Part model, mm, in its own coordinate system. Coordinates: 2 decimals unless noted, no trailing zeros. Loops run counter-clockwise (first coordinate to the right, second up) from the corner with the lowest first, then second, coordinate; pieces in that order, holes last. Notation, with made-up numbers: M 82,-1 L 140,-1 A25 cw 140,32 Z; hole C 20.25,80.25 d5. An arc over 180 degrees is marked long. Use a Markdown table: item, result. Add a question column.
1) Wall check: probe 1 along X at (y, z) = (1.9, -43); probe 2 along X at (y, z) = (0.25, -67); probe 3 along X at (y, z) = (1.95, -62). Give the ranges that are in metal, low to high. Write a range as from..to.
2) Band-saw the part on D-D (z = -54.5). List the corners of the cut face in (x, y), plus the area to 3 significant figures.
3) Band-saw the part on A-A (z = -43). List the corners of the cut face in (x, y).
4) Pin check, flat tips, straight feed: pin 1 Ø1 at (x, z) = (-24.5, -54) entering from -Y; pin 2 Ø4 at (x, z) = (0, -65) entering from -Y. Stop position of each tip, or through.
5) Band-saw the part on C-C (y = 2.05). List the corners of the cut face in (x, z).
6) Band-saw the part on B-B (x = 0). List the corners of the cut face in (y, z), plus the area to 3 significant figures.
from build123d import *

# Parameters (mm, degrees)
BOSS_EXTRUDE1_DEPTH  = 3
CUT_EXTRUDE14_DEPTH  = 103.574363269
SKETCH14_OUTSIDE_W   = 186.736
SKETCH14_OUTSIDE_H   = 177.534
SKETCH14_OUTSIDE_W_2 = 80
SKETCH14_OUTSIDE_H_2 = 40
CUT_EXTRUDE15_DEPTH  = 103.574363269
SKETCH15_R           = 2.4
CUT_EXTRUDE16_DEPTH  = 83.856804186


with BuildPart() as part:
    # Sketch1 → Boss-Extrude1 (new body)
    with BuildSketch(Plane(origin=(0, 0, 0), x_dir=(1, 0, 0), z_dir=(0, 1, 0))):
        with BuildLine():
            ThreePointArc((36.543377003, -62.616544118), (0, 72.5), (-36.543377003, -62.616544118))
            ThreePointArc((-36.543377003, -62.616544118), (-33.085954668, -63.20954405), (-30.089832649, -61.38507948))
            ThreePointArc((-30.089832649, -61.38507948), (0, -46.75), (30.089832649, -61.38507948))
            ThreePointArc((30.089832649, -61.38507948), (33.085954668, -63.20954405), (36.543377003, -62.616544118))
        make_face()
    extrude(amount=BOSS_EXTRUDE1_DEPTH)

    # Sketch13 → Cut-Extrude14 (cut, through all)
    with BuildSketch(Plane(origin=(0, 3, 0), x_dir=(1, 0, 0), z_dir=(0, 1, 0))):
        with BuildLine():
            Line((-9.638836445, 48.2), (9.638836445, 48.2))
            ThreePointArc((9.638836445, 48.2), (10.961172041, 48.699523885), (11.622969422, 49.948571429))
            ThreePointArc((11.622969422, 49.948571429), (13.054510917, 54.765599326), (15.951885484, 58.871484058))
            ThreePointArc((15.951885484, 58.871484058), (16.449270482, 60.8240474), (14.994913363, 62.21858704))
            ThreePointArc((14.994913363, 62.21858704), (12.303854546, 62.806171379), (9.590005203, 63.277419355))
            ThreePointArc((9.590005203, 63.277419355), (8.295362524, 63.03495375), (7.432254032, 62.04))
            ThreePointArc((7.432254032, 62.04), (0, 57), (-7.432254032, 62.04))
            ThreePointArc((-7.432254032, 62.04), (-8.295362524, 63.03495375), (-9.590005203, 63.277419355))
            ThreePointArc((-9.590005203, 63.277419355), (-12.303854546, 62.806171379), (-14.994913363, 62.21858704))
            ThreePointArc((-14.994913363, 62.21858704), (-16.449270482, 60.8240474), (-15.951885484, 58.871484058))
            ThreePointArc((-15.951885484, 58.871484058), (-13.054510917, 54.765599326), (-11.622969422, 49.948571429))
            ThreePointArc((-11.622969422, 49.948571429), (-10.961172041, 48.699523885), (-9.638836445, 48.2))
        make_face()
    extrude(amount=-CUT_EXTRUDE14_DEPTH, mode=Mode.SUBTRACT)

    # Sketch14 outside → Cut-Extrude15 (cut, through all)
    with BuildSketch(Plane(origin=(0, 3, 0), x_dir=(1, 0, 0), z_dir=(0, 1, 0))):
        with Locations((0, 4.601)):
            Rectangle(SKETCH14_OUTSIDE_W, SKETCH14_OUTSIDE_H)
        with Locations((0, 57)):
            Rectangle(SKETCH14_OUTSIDE_W_2, SKETCH14_OUTSIDE_H_2, mode=Mode.SUBTRACT)
    extrude(amount=-CUT_EXTRUDE15_DEPTH, mode=Mode.SUBTRACT)

    # Sketch15 → Cut-Extrude16 (cut, through all)
    with BuildSketch(Plane(origin=(0, 3, 0), x_dir=(1, 0, 0), z_dir=(0, 1, 0))):
        with Locations(Location((0, 65, 0), (0, 0, 270))):
            Circle(SKETCH15_R)
        with Locations(Location((0, 43, 0), (0, 0, 270))):
            Circle(SKETCH15_R)
    extrude(amount=-CUT_EXTRUDE16_DEPTH, mode=Mode.SUBTRACT)


solid = part.part
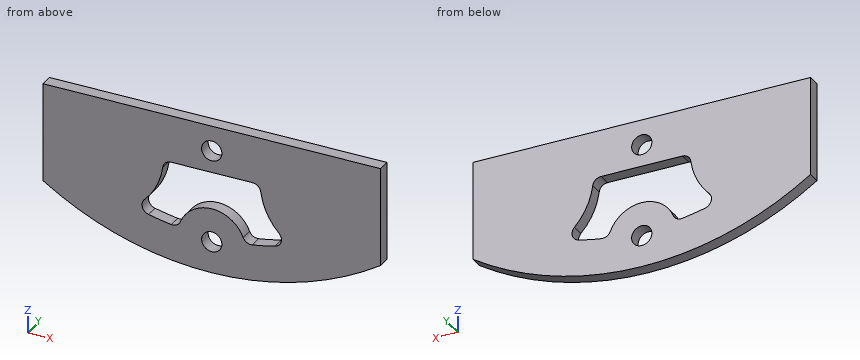
Entries:
| question | item | result |
|---|---|---|
| 1 | probe 1 | -40..-2.4, 2.4..40 |
| 1 | probe 2 | -27.7..-1.33, 1.33..27.7 |
| 1 | probe 3 | -37.58..-15.54, -7.42..7.42, 15.54..37.58 |
| 2 | outline | M -40,0 L -12.93,0 L -12.93,3 L -40,3 Z; M 12.93,0 L 40,0 L 40,3 L 12.93,3 Z |
| 2 | area | 162 mm2 |
| 3 | outline | M -40,0 L -2.4,0 L -2.4,3 L -40,3 Z; M 2.4,0 L 40,0 L 40,3 L 2.4,3 Z |
| 4 | pin 1 | y = 0 |
| 4 | pin 2 | through |
| 5 | outline | M -40,-60.47 A72.5 ccw 40,-60.47 L 40,-37 L -40,-37 Z; hole M -15.95,-58.87 A2 ccw -14.99,-62.22 A64 ccw -9.59,-63.28 A2 ccw -7.43,-62.04 A8 cw 7.43,-62.04 A2 ccw 9.59,-63.28 A64 ccw 14.99,-62.22 A2 ccw 15.95,-58.87 A15.5 cw 11.62,-49.95 A2 ccw 9.64,-48.2 L -9.64,-48.2 A2 ccw -11.62,-49.95 A15.5 cw Z; hole C 0,-65 d4.8; hole C 0,-43 d4.8 |
| 6 | outline | M 0,-72.5 L 3,-72.5 L 3,-67.4 L 0,-67.4 Z; M 0,-62.6 L 3,-62.6 L 3,-57 L 0,-57 Z; M 0,-48.2 L 3,-48.2 L 3,-45.4 L 0,-45.4 Z; M 0,-40.6 L 3,-40.6 L 3,-37 L 0,-37 Z |
| 6 | area | 51.3 mm2 |
